Source: three-view drawing plus pictorial views. Frame: mm from the lowest corner of the part. A direction names the side the tool comes from. Give positions to 0.01 mm unless a question says otherwise; leave off trailing zeros. Order: outer loops, then holes, each group sorted by start corner. A loop starts at its lowest first (then second) coordinate and runs counter-clockwise, first axis right, second up. Notation, with made-up numbers: (42.5, -7.5) - (70.5, -7.5) arc R38 ccw to (70.5, 30.5) - close; hole circle Ø2 at (86.5, 0). An arc over 180 degrees is marked (long way). Use CSV: the item, a comma, the result in double quotes.
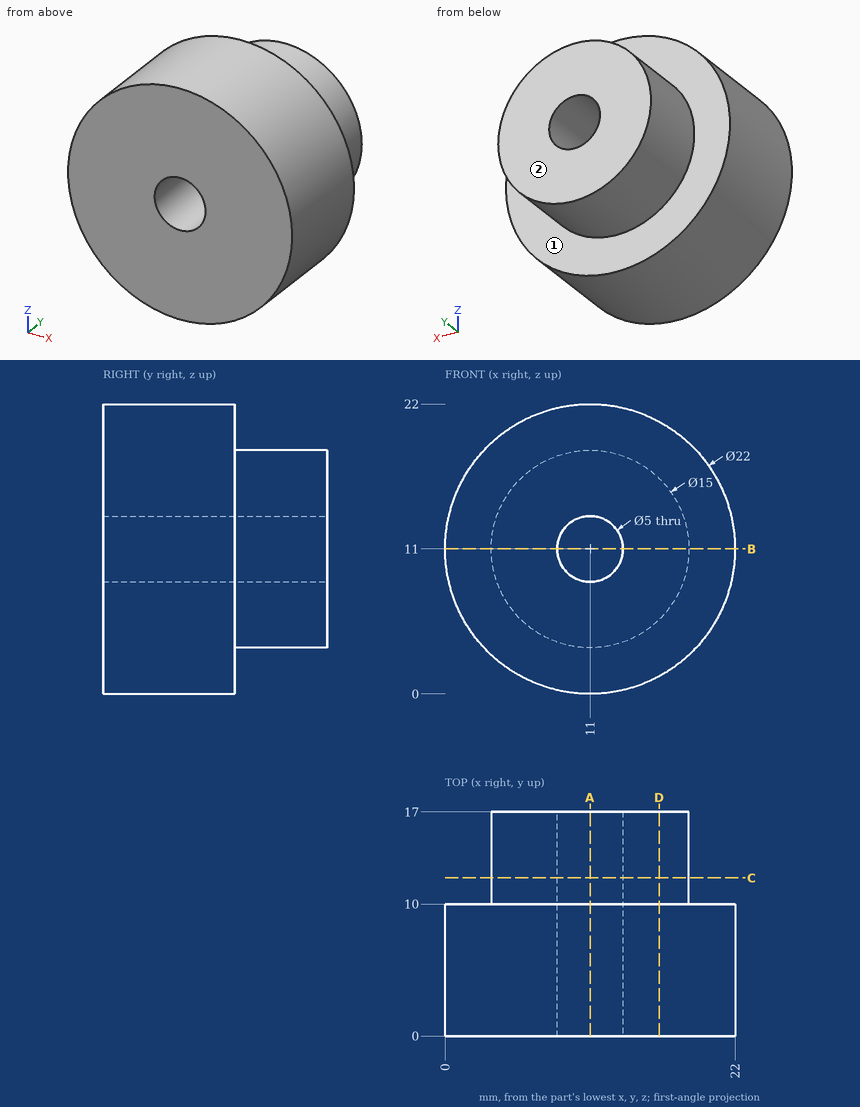
Item 1: Section D-D on x = 16.25. Return the cut outline in (y, z).
Filled in:
outline,"(0, 1.33) - (10, 1.33) - (10, 5.64) - (17, 5.64) - (17, 16.36) - (10, 16.36) - (10, 20.67) - (0, 20.67) - close"
Item 2: Section B-B on z = 11. Return the cut outline in (x, y).
Filled in:
outline,"(0, 0) - (8.5, 0) - (8.5, 17) - (3.5, 17) - (3.5, 10) - (0, 10) - close; (13.5, 0) - (22, 0) - (22, 10) - (18.5, 10) - (18.5, 17) - (13.5, 17) - close"
Item 3: First-contact query: pin 1 (10 mm diameter, centred on x = 12.5, y = 13, fed in from -Z); pin 2 (5 mm diameter, centred on x = 15.5, y = 3, fed in from -Z); pin 3 (1.5 mm diameter, centred on y = 12, z = 15, fed in from -X); pin 4 (10 mm diameter, centred on y = 3.5, z = 3, fed in from +X). Flat tips, straight axial feed; report the tip coordinate or a pass-through.
Filled in:
pin 1,"stops at z = 0"
pin 2,"stops at z = 0.18"
pin 3,"stops at x = 4.24"
pin 4,"stops at x = 21.58"
Item 4: Section C-C on y = 12. Return the cut outline in (x, z).
Filled in:
outline,"circle Ø15 at (11, 11); hole circle Ø5 at (11, 11)"
Item 5: Material intervals for line 1 (X direction, y = 4, z = 11); line 2 (Z direction, x = 11, y = 12.25), sorted ascending. Write a range as from..to.
Filled in:
line 1,"x = 0..8.5, 13.5..22"
line 2,"z = 3.5..8.5, 13.5..18.5"
Item 6: Section A-A on x = 11. Return the cut outline in (y, z).
Filled in:
outline,"(0, 0) - (10, 0) - (10, 3.5) - (17, 3.5) - (17, 8.5) - (0, 8.5) - close; (0, 13.5) - (17, 13.5) - (17, 18.5) - (10, 18.5) - (10, 22) - (0, 22) - close"
Item 7: Set-up query: the marked faces 1 and 2. Return all of +Z, -Z, +X, -X, +Y, -Y with unobstructed straight access to the full face (end or side cutting, diameter ignored); none if empty.
Filled in:
face 1,"+Y"
face 2,"+Z, -Z, +X, -X, +Y"
